from build123d import *

# Parameters (mm, degrees)
SKETCH2_W                 = 50.8
SKETCH2_H                 = 92.075
BOSS_EXTRUDE1_DEPTH       = 6.35
SKETCH3_W                 = 51.30062604
SKETCH3_H                 = 6.35
BOSS_EXTRUDE2_DEPTH       = 88.9
FILLET1_R                 = 9.8425
SKETCH4_W                 = 50.8
SKETCH4_H                 = 6.35
BOSS_EXTRUDE3_DEPTH       = 38.1
SKETCH7_W                 = 19.05
SKETCH7_H                 = 9.525
BOSS_EXTRUDE4_DEPTH       = 92.075
BOSS_EXTRUDE7_START       = -7.62
SKETCH5_R                 = 9.525
SKETCH5_R_2               = 4.7625
BOSS_EXTRUDE7_DEPTH       = 11.43
BOSS_EXTRUDE8_START       = 7.62
BOSS_EXTRUDE8_DEPTH       = 11.43
SKETCH11_W                = 11.43
SKETCH11_H                = 9.525
BOSS_EXTRUDE9_DEPTH       = 2.425484171
BOSS_EXTRUDE10_DEPTH      = 6.35
BOSS_EXTRUDE10_DEPTH_BACK = 6.35
BOSS_EXTRUDE11_START      = 6.35
BOSS_EXTRUDE11_DEPTH      = 6.35
BOSS_EXTRUDE12_START      = -12.7
BOSS_EXTRUDE12_DEPTH      = 6.35
BOSS_EXTRUDE13_START      = -34.925
SKETCH18_W                = 50.8
SKETCH18_H                = 6.35
BOSS_EXTRUDE13_DEPTH      = 76.2
SKETCH17_R                = 3.657298314
CUT_EXTRUDE4_DEPTH        = 6.35
CUT_EXTRUDE5_DEPTH        = 6.35
BOSS_EXTRUDE14_DEPTH      = 6.35
BOSS_EXTRUDE14_DEPTH_BACK = 6.35
FILLET2_R                 = 12.7
FILLET3_R                 = 3.175


with BuildPart() as part:
    # Sketch2 → Boss-Extrude1 (new body)
    with BuildSketch(Plane(origin=(0, 0, 0), x_dir=(1, 0, 0), z_dir=(0, 1, 0))):
        with Locations((25.4, 46.0375)):
            Rectangle(SKETCH2_W, SKETCH2_H)
    extrude(amount=BOSS_EXTRUDE1_DEPTH)

    # Sketch3 → Boss-Extrude2 (add)
    with BuildSketch(Plane(origin=(0, 6.35, 0), x_dir=(1, 0, 0), z_dir=(0, 1, 0))):
        with Locations((25.14968698, 38.1)):
            Rectangle(SKETCH3_W, SKETCH3_H)
    extrude(amount=BOSS_EXTRUDE2_DEPTH)

    # Fillet1
    fillet1_edges = [part.edges().sort_by_distance(p)[0] for p in [
        (25.4, 6.35, -34.925),
    ]]
    fillet(fillet1_edges, radius=FILLET1_R)

    # Sketch4 → Boss-Extrude3 (add)
    with BuildSketch(Plane(origin=(0, 0, -92.075), x_dir=(-1, 0, 0), z_dir=(0, 0, -1))):
        with Locations((-25.4, 3.175)):
            Rectangle(SKETCH4_W, SKETCH4_H)
    extrude(amount=BOSS_EXTRUDE3_DEPTH)

    # Sketch7 → Boss-Extrude4 (add)
    with BuildSketch(Plane(origin=(0, 0, 0), x_dir=(-1, 0, 0), z_dir=(0, -1, 0))):
        with Locations((-15.875, 125.4125)):
            Rectangle(SKETCH7_W, SKETCH7_H)
        with Locations((-34.925, 125.4125)):
            Rectangle(SKETCH7_W, SKETCH7_H)
    extrude(amount=BOSS_EXTRUDE4_DEPTH)



with BuildPart() as body_2:
    # Sketch5 → Boss-Extrude7 (new body)
    with BuildSketch(Plane(origin=(25.4, 0, 0), x_dir=(0, 0, -1), z_dir=(1, 0, 0)).offset(BOSS_EXTRUDE7_START)):
        with Locations((127, -101.6)):
            Circle(SKETCH5_R)
        with Locations((127, -101.6)):
            Circle(SKETCH5_R_2, mode=Mode.SUBTRACT)
    extrude(amount=-BOSS_EXTRUDE7_DEPTH)


with BuildPart() as body_3:
    # Sketch5<6> → Boss-Extrude8 (new body)
    with BuildSketch(Plane(origin=(25.4, 0, 0), x_dir=(0, 0, -1), z_dir=(1, 0, 0)).offset(BOSS_EXTRUDE8_START)):
        with BuildLine():
            ThreePointArc((127, -92.075), (120.264807909, -94.864807909), (117.475, -101.6))
            Line((117.475, -101.6), (122.2375, -101.6))
            ThreePointArc((122.2375, -101.6), (123.632403955, -98.232403955), (127, -96.8375))
            Line((127, -96.8375), (127, -92.075))
        make_face()
        with BuildLine():
            Line((122.2375, -101.6), (117.475, -101.6))
            ThreePointArc((117.475, -101.6), (127, -111.125), (136.525, -101.6))
            ThreePointArc((136.525, -101.6), (133.735192091, -94.864807909), (127, -92.075))
            Line((127, -92.075), (127, -96.8375))
            ThreePointArc((127, -96.8375), (130.367596045, -98.232403955), (131.7625, -101.6))
            ThreePointArc((131.7625, -101.6), (127, -106.3625), (122.2375, -101.6))
        make_face()
    extrude(amount=BOSS_EXTRUDE8_DEPTH)


with BuildPart() as part_1:
    add(part.part)

    add(body_2.part)  # Boss-Extrude9 merges body 2

    add(body_3.part)  # Boss-Extrude9 merges body 3
    # Sketch11 → Boss-Extrude9 (add)
    with BuildSketch(Plane.XZ.offset(92.075)):
        with Locations((12.065, -125.4125)):
            Rectangle(SKETCH11_W, SKETCH11_H)
        with Locations((38.735, -125.4125)):
            Rectangle(SKETCH11_W, SKETCH11_H)
    extrude(amount=BOSS_EXTRUDE9_DEPTH)

    # Sketch13 → Boss-Extrude10 (add, two sides: drawn at the far end of the back side and taken through both)
    with BuildSketch(Plane(origin=(25.4, 0, 0), x_dir=(0, 0, -1), z_dir=(1, 0, 0)).offset(-BOSS_EXTRUDE10_DEPTH_BACK)):
        Polygon((120.65, -79.375), (41.275, 0), (28.575, 0), (120.65, -92.075), align=None)
    extrude(amount=BOSS_EXTRUDE10_DEPTH + BOSS_EXTRUDE10_DEPTH_BACK)

    # Sketch15 → Boss-Extrude11 (add)
    with BuildSketch(Plane(origin=(25.4, 0, 0), x_dir=(0, 0, -1), z_dir=(1, 0, 0)).offset(BOSS_EXTRUDE11_START)):
        with BuildLine():
            ThreePointArc((12.7, -6.35), (10.840128061, -1.859871939), (6.35, 0))
            ThreePointArc((6.35, 0), (1.859871939, -1.859871939), (0, -6.35))
            Line((0, -6.35), (3.175, -6.35))
            ThreePointArc((3.175, -6.35), (6.35, -3.175), (9.525, -6.35))
            Line((9.525, -6.35), (12.7, -6.35))
        make_face()
        with BuildLine():
            Line((3.175, -6.35), (0, -6.35))
            ThreePointArc((0, -6.35), (6.35, -12.7), (12.7, -6.35))
            Line((12.7, -6.35), (9.525, -6.35))
            ThreePointArc((9.525, -6.35), (6.35, -9.525), (3.175, -6.35))
        make_face()
        with BuildLine():
            Line((6.35, 0), (0, 0))
            Line((0, 0), (0, -6.35))
            ThreePointArc((0, -6.35), (1.859871939, -1.859871939), (6.35, 0))
        make_face()
        with BuildLine():
            Line((12.7, 0), (6.35, 0))
            ThreePointArc((6.35, 0), (10.840128061, -1.859871939), (12.7, -6.35))
            Line((12.7, -6.35), (12.7, 0))
        make_face()
    extrude(amount=BOSS_EXTRUDE11_DEPTH)

    # Sketch15<3> → Boss-Extrude12 (add)
    with BuildSketch(Plane(origin=(25.4, 0, 0), x_dir=(0, 0, -1), z_dir=(1, 0, 0)).offset(BOSS_EXTRUDE12_START)):
        with BuildLine():
            ThreePointArc((12.7, -6.35), (10.840128061, -1.859871939), (6.35, 0))
            ThreePointArc((6.35, 0), (1.859871939, -1.859871939), (0, -6.35))
            Line((0, -6.35), (3.175, -6.35))
            ThreePointArc((3.175, -6.35), (6.35, -3.175), (9.525, -6.35))
            Line((9.525, -6.35), (12.7, -6.35))
        make_face()
        with BuildLine():
            Line((3.175, -6.35), (0, -6.35))
            ThreePointArc((0, -6.35), (6.35, -12.7), (12.7, -6.35))
            Line((12.7, -6.35), (9.525, -6.35))
            ThreePointArc((9.525, -6.35), (6.35, -9.525), (3.175, -6.35))
        make_face()
        with BuildLine():
            Line((6.35, 0), (0, 0))
            Line((0, 0), (0, -6.35))
            ThreePointArc((0, -6.35), (1.859871939, -1.859871939), (6.35, 0))
        make_face()
        with BuildLine():
            Line((12.7, 0), (6.35, 0))
            ThreePointArc((6.35, 0), (10.840128061, -1.859871939), (12.7, -6.35))
            Line((12.7, -6.35), (12.7, 0))
        make_face()
    extrude(amount=BOSS_EXTRUDE12_DEPTH)

    # Sketch18 → Boss-Extrude13 (add)
    with BuildSketch(Plane.XY.offset(BOSS_EXTRUDE13_START)):
        with Locations((25.4, 3.175)):
            Rectangle(SKETCH18_W, SKETCH18_H)
    extrude(amount=BOSS_EXTRUDE13_DEPTH)

    # Sketch17 → Cut-Extrude4 (cut)
    with BuildSketch(Plane(origin=(0, 0, 0), x_dir=(-1, 0, 0), z_dir=(0, -1, 0))):
        with Locations(Location((-44.45, 19.05, 0), (0, 0, 90))):
            Circle(SKETCH17_R)
        with Locations(Location((-6.35, 19.05, 0), (0, 0, 90))):
            Circle(SKETCH17_R)
    extrude(amount=-CUT_EXTRUDE4_DEPTH, mode=Mode.SUBTRACT)

    # Sketch19 → Cut-Extrude5 (cut)
    with BuildSketch(Plane(origin=(0, 0, -41.275), x_dir=(-1, 0, 0), z_dir=(0, 0, -1))):
        with BuildLine():
            ThreePointArc((-28.32468698, 88.9), (-25.14968698, 85.725), (-21.97468698, 88.9))
            Line((-21.97468698, 88.9), (-28.32468698, 88.9))
        make_face()
        with BuildLine():
            Line((-28.32468698, 88.9), (-21.97468698, 88.9))
            ThreePointArc((-21.97468698, 88.9), (-25.14968698, 92.075), (-28.32468698, 88.9))
        make_face()
    extrude(amount=-CUT_EXTRUDE5_DEPTH, mode=Mode.SUBTRACT)

    # Sketch20 → Boss-Extrude14 (add, two sides: drawn at the far end of the back side and taken through both)
    with BuildSketch(Plane(origin=(25.4, 0, 0), x_dir=(0, 0, -1), z_dir=(1, 0, 0)).offset(-BOSS_EXTRUDE14_DEPTH_BACK)):
        Polygon((41.275, 82.55), (130.175, 6.35), (120.417648783, 6.35), (41.275, 74.186556099), align=None)
    extrude(amount=BOSS_EXTRUDE14_DEPTH + BOSS_EXTRUDE14_DEPTH_BACK)

    # Fillet2
    fillet2_edges = [part_1.edges().sort_by_distance(p)[0] for p in [
        (25.4, 0, -120.65),
    ]]
    fillet(fillet2_edges, radius=FILLET2_R)

    # Fillet3
    # the kernel refuses this fillet: 3.175 mm, written as the material it adds along each edge
    with BuildSketch(Plane(origin=(33.02, -92.075, -120.65), x_dir=(-1, 0, 0), z_dir=(0, 0, -1))) as fillet3_piece_1:
        with BuildLine():
            CenterArc((FILLET3_R, -FILLET3_R), FILLET3_R, 90, 90)
            Line((0, -FILLET3_R), (0, 0))
            Line((0, 0), (FILLET3_R, 0))
        make_face()
    extrude(amount=9.525)
    with BuildSketch(Plane(origin=(33.02, -92.075, -112.7125), x_dir=(-1, 0, 0), z_dir=(0, 0, -1))) as fillet3_piece_2_section:
        with BuildLine():
            CenterArc((FILLET3_R, -FILLET3_R), FILLET3_R, 90, 90)
            Line((0, -FILLET3_R), (0, 0))
            Line((0, 0), (FILLET3_R, 0))
        make_face()
    fillet3_piece_2 = extrude(amount=25.4, mode=Mode.PRIVATE)
    fillet3_piece_2 = fillet3_piece_2 & Plane(origin=(33.001906898, -101.6, -127), x_dir=(0, 1, 0), z_dir=(-1, 0, 0)) * Cylinder(9.525, 64, mode=Mode.PRIVATE)
    add(fillet3_piece_2)
    with BuildSketch(Plane(origin=(17.78, -92.075, -120.65), x_dir=(1, 0, 0), z_dir=(0, 0, -1))) as fillet3_piece_3:
        with BuildLine():
            CenterArc((FILLET3_R, FILLET3_R), FILLET3_R, 180, 90)
            Line((0, FILLET3_R), (0, 0))
            Line((0, 0), (FILLET3_R, 0))
        make_face()
    extrude(amount=9.525)
    with BuildSketch(Plane(origin=(17.78, -92.075, -112.7125), x_dir=(1, 0, 0), z_dir=(0, 0, -1))) as fillet3_piece_4_section:
        with BuildLine():
            CenterArc((FILLET3_R, FILLET3_R), FILLET3_R, 180, 90)
            Line((0, FILLET3_R), (0, 0))
            Line((0, 0), (FILLET3_R, 0))
        make_face()
    fillet3_piece_4 = extrude(amount=25.4, mode=Mode.PRIVATE)
    fillet3_piece_4 = fillet3_piece_4 & Plane(origin=(17.798093102, -101.6, -127), x_dir=(0, 0, -1), z_dir=(1, 0, 0)) * Cylinder(9.525, 64, mode=Mode.PRIVATE)
    add(fillet3_piece_4)


solid = part_1.part
Work out the finished part from the listing and answer in its coordinate system (mm). A direction names the side the tool comes from. Give positions to 0.01 mm unless a question says otherwise; leave off trailing zeros. Loops run counter-clockwise (first coordinate to the right, second up) from the corner with the lowest first, then second, coordinate; pieces in that order, holes last. Notation, with made-up numbers: (12.25, -33) -> (31.25, -33) arc R33 cw to (31.25, 5) -> close; hole circle Ø11 at (71, -7.5). An arc over 180 degrees is marked (long way). Use a Markdown table: item, result. Add a question column.
1. Section C-C on z = -111 is taken. Determine the outline of the cut face in (x, y) (3 decimals), and give its area (3 significant figures).
2. Determine the mould class of faces 5 (the flat face through (31.75, 42, -83)), 6 (the cylindrical face through (12.853, -111.006, -128.503)), 7 (the flat face through (25.311, -45.393, -73.968)), 8 (the flat face through (16, -3, -12.7)) for opening direction Z: released by +Z, released by -Z, zero draft, split by the parting line, or undercut.
3. For faces 1 (the flat face through (38.1, -3, -8)), 2 (the flat face through (33.02, -107, -127)), 3 (the flat face through (19.05, -42, -78)), 4 (the flat face through (16, -3, 0)), determine the directions among +Z, -Z, +X, -X, +Y, -Y from which every point of the face is accessible in a straight line to the end or side of a thin tool.
4. Find the intervals of material crossed by probe 1 along Y at (x, z) = (33.5, -6.35) (3 decimals); probe 2 along Y at (x, z) = (25, -67) (3 decimals); probe 3 along Y at (x, z) = (28, -59.5) (3 decimals), in increasing order.
5. Flat-ended cylindrical pins translate along their axes: pin 1 Ø15 at (x, z) = (18.5, -6.5) entering from +Y; pin 2 Ø10 at (x, z) = (31, -45) entering from -Y (3 decimals); pin 3 Ø5 at (x, z) = (23.5, -61.5) entering from -Y (3 decimals). Find the tip coordinate at first contact, or state that the pin passes through.
6. Section A-A on y = 88.9 is taken. Determine the outline of the cut face in (x, z) (3 decimals).
7. Section D-D on y = 50 is taken. Determine the outline of the cut face in (x, z) (3 decimals), and give its area (3 significant figures).
8. Section B-B on z = -19.05 is taken. Determine the outline of the cut face in (x, y).
Results below:
| question | item | result |
|---|---|---|
| 1 | outline | (0, 0) -> (6.35, 0) -> (6.35, -0.372) -> (44.45, -0.372) -> (44.45, 0) -> (50.8, 0) -> (50.8, 6.35) -> (0, 6.35) -> close; (19.05, -82.425) -> (31.75, -82.425) -> (31.75, -69.725) -> (19.05, -69.725) -> close; (19.05, 14.422) -> (31.75, 14.422) -> (31.75, 22.786) -> (19.05, 22.786) -> close |
| 1 | area | 604 mm^2 |
| 2 | face 5 | zero draft |
| 2 | face 6 | split by the parting line |
| 2 | face 7 | released by +Z |
| 2 | face 8 | undercut |
| 3 | face 1 | +Z, +X, -Y |
| 3 | face 2 | +Z, -Z, -Y |
| 3 | face 3 | -X, -Y |
| 3 | face 4 | +Z, +X, -X, -Y |
| 4 | probe 1 | y = -12.7 to -9.525, -3.175 to 6.35 |
| 4 | probe 2 | y = -38.425 to -25.725, 0 to 6.35, 52.137 to 60.5 |
| 4 | probe 3 | y = -30.925 to -18.225, 0 to 6.35, 58.565 to 66.929 |
| 5 | pin 1 | stops at y = 6.35 |
| 5 | pin 2 | stops at y = -21.425 |
| 5 | pin 3 | stops at y = -35.425 |
| 6 | outline | (-0.501, -41.275) -> (21.975, -41.275) -> (21.975, -34.925) -> (-0.501, -34.925) -> close; (28.325, -41.275) -> (50.8, -41.275) -> (50.8, -34.925) -> (28.325, -34.925) -> close |
| 7 | outline | (-0.501, -41.275) -> (50.8, -41.275) -> (50.8, -34.925) -> (-0.501, -34.925) -> close; (19.05, -79.25) -> (31.75, -79.25) -> (31.75, -69.493) -> (19.05, -69.493) -> close |
| 7 | area | 450 mm^2 |
| 8 | outline | (0, 0) -> (2.69, 0) -> (2.69, 6.35) -> (0, 6.35) -> close; (10.01, 0) -> (40.79, 0) -> (40.79, 6.35) -> (10.01, 6.35) -> close; (48.11, 0) -> (50.8, 0) -> (50.8, 6.35) -> (48.11, 6.35) -> close |
